Job drawing, mm, ordinate dimensions from the low corner. One solid piece. Give positions to 0.01 mm unless a question says otherwise; leave off trailing zeros. Write each loop counter-clockwise with the first axis right and the second up, starting at its lowest first coordinate (ties: lowest second). Pieces come first, ordered by that corner, then holes. Notation, with made-up numbers: M 79,65 L 101,65 A17 ccw 101,79 Z; hole C -12.75,-3.75 d5. An arc over 180 degrees is marked long. Use CSV: the item, a comma, the result in double quotes. Start each with the question number.
Item 1: Cut at A-A (y = 13.75). List the corners of the cut face in (x, z).
Item 2: Pin check, flat tip, straight feed: pin 1 (3 mm diameter, centred on x = 5, y = 9, fed in from -Z). Stop position of the tip, or through.
Item 3: Drill centre lines: line 1 (Y direction, x = 16.75, z = 1.9); line 2 (Y direction, x = 14.5, z = 1.4); line 3 (X direction, y = 17.5, z = 0.55) (1 decimal). Where is each one in solid material? Low to high. Write a range as [from, to].
Item 4: Cut at B-B (x = 18). List the corners of the cut face in (y, z).
Item 5: Cut at C-C (z = 1.3). List the corners of the cut face in (x, y).
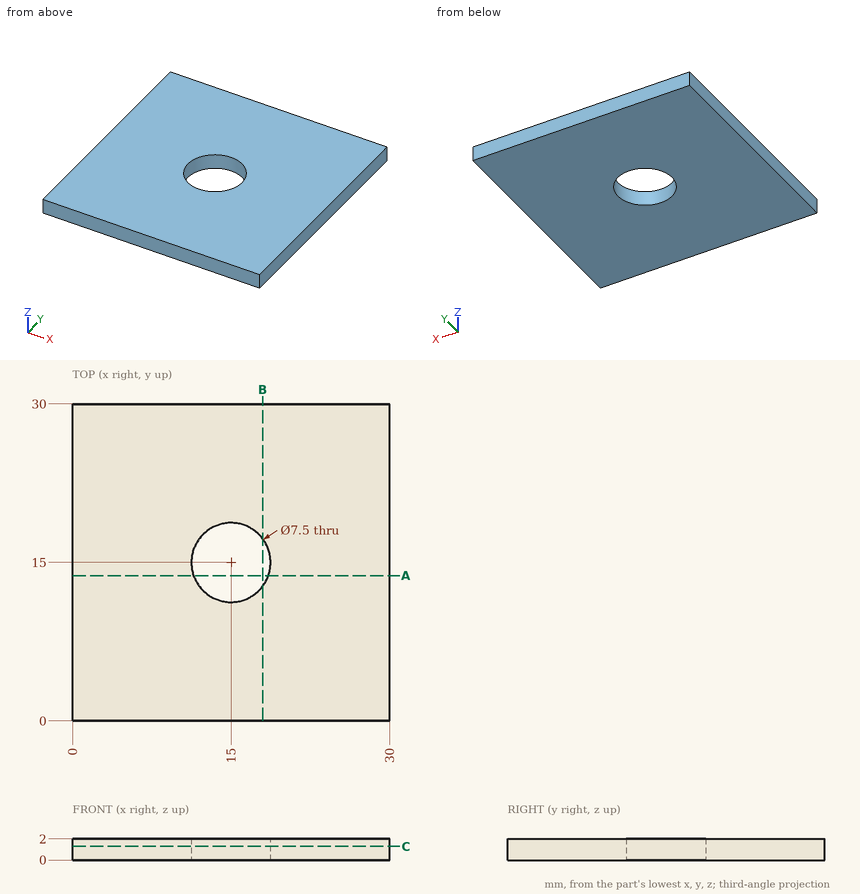
Worked answers:
1,outline,"M 0,0 L 11.46,0 L 11.46,2 L 0,2 Z; M 18.54,0 L 30,0 L 30,2 L 18.54,2 Z"
2,pin 1,"stops at z = 0"
3,line 1,"y = [0, 11.68], [18.32, 30]"
3,line 2,"y = [0, 11.28], [18.72, 30]"
3,line 3,"x = [0, 12.2], [17.8, 30]"
4,outline,"M 0,0 L 12.75,0 L 12.75,2 L 0,2 Z; M 17.25,0 L 30,0 L 30,2 L 17.25,2 Z"
5,outline,"M 0,0 L 30,0 L 30,30 L 0,30 Z; hole C 15,15 d7.5"
